from build123d import *

# Parameters (mm, degrees)
EXTRUDE_1_DEPTH     = 46
SKETCH_2_R          = 6
CUT_EXTRUDE_1_DEPTH = 45


with BuildPart() as part:
    # ｽｹｯﾁ1 → ﾎﾞｽ - 押し出し1 (new body)
    with BuildSketch(Plane.XY):
        with BuildLine():
            Line((-9.5, 0), (-7.25, 0))
            ThreePointArc((-7.25, 0), (0, 7.25), (7.25, 0))
            Line((7.25, 0), (9.5, 0))
            ThreePointArc((9.5, 0), (0, 9.5), (-9.5, 0))
        make_face()
    extrude(amount=EXTRUDE_1_DEPTH)

    # ｽｹｯﾁ2 → ｶｯﾄ - 押し出し1 (cut)
    with BuildSketch(Plane(origin=(0, 0, 0), x_dir=(1, 0, 0), z_dir=(0, 1, 0))):
        with Locations(Location((0, -22.5, 0), (0, 0, 90))):
            Circle(SKETCH_2_R)
    extrude(amount=CUT_EXTRUDE_1_DEPTH, mode=Mode.SUBTRACT)


solid = part.part
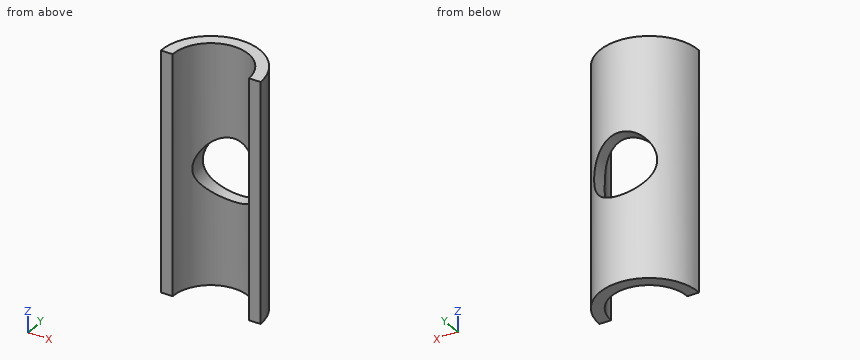
Source: CAD feature listing. Evaluate the final solid. Frame: model axes, mm. Round coordinates to 2 decimals unless told otherwise and drop trailing zeros. Loops run counter-clockwise (first coordinate to the right, second up) from the corner with the lowest first, then second, coordinate; pieces in that order, holes last. Notation, with made-up numbers: M 1,6 L 53,6 A27 cw 53,37 Z; hole C 8.5,17.25 d9. An arc over 180 degrees is marked long. Return JSON: item names as keys, results as strings. Group by question number.
1. Material intervals for line 1 along X through (y, z) = (6.15, 22.5); line 2 along X through (y, z) = (2.75, 35); line 3 along Z through (x, y) = (2.75, 6.75), sorted ascending. Write a range as from..to.
2. Section query A-A on x = 0. Output: boundary loops of the cut face in (y, z).
3. Pin query (flat end, axial travel): pin 1 (4 mm diameter, centred on x = -1, z = 41, fed in from -Y); pin 2 (1.5 mm diameter, centred on x = 5, z = 40, fed in from +Y); pin 3 (3 mm diameter, centred on x = -0.5, z = 31.5, fed in from -Y); pin 4 (1 mm diameter, centred on x = -5.5, y = 7, fed in from -Z). Return the tip coordinate at first contact, or that it passes through.
4. Section query B-B on y = 7.75. Output: boundary loops of the cut face in (x, z).
5. Section query C-C on z = 3. Output: boundary loops of the cut face in (x, y).
6. Section query D-D on x = 8.25. Output: boundary loops of the cut face in (y, z), and give its area (3 significant figures).
Checks:
{
 "1": {"line 1": "x = -7.24..-6, 6..7.24", "line 2": "x = -9.09..-6.71, 6.71..9.09", "line 3": "z = 0..17.17, 27.83..46"},
 "2": {"outline": "M 7.25,0 L 9.5,0 L 9.5,16.5 L 7.25,16.5 Z; M 7.25,28.5 L 9.5,28.5 L 9.5,46 L 7.25,46 Z"},
 "3": {"pin 1": "stops at y = 6.6", "pin 2": "stops at y = 8.5", "pin 3": "stops at y = 6.97", "pin 4": "stops at z = 0"},
 "4": {"outline": "M -5.49,0 L 5.49,0 L 5.49,20.09 A6 cw -5.49,20.09 Z; M -5.49,24.91 A6 cw 5.49,24.91 L 5.49,46 L -5.49,46 Z"},
 "5": {"outline": "M -9.5,0 L -7.25,0 A7.25 cw 7.25,0 L 9.5,0 A9.5 ccw Z"},
 "6": {"outline": "M 0,0 L 4.71,0 L 4.71,46 L 0,46 Z", "area": "217 mm²"}
}
